Read the model definition and answer for the solid it produces. Units are mm, in the model's axes. Face numbers are marked on the shaded views. Give positions to 0.01 mm unless a question says otherwise; leave off trailing zeros. Order: outer loops, then holes, each group sorted by start corner. A loop starts at its lowest first (then second) coordinate and runs counter-clockwise, first axis right, second up. Notation, with made-up numbers: (12.25, -36) - (71.25, -36) arc R24 ccw to (71.25, -21) - close; hole circle Ø7 at (26.25, 82.5). An arc over 180 degrees is marked (long way). One line per item, written item: value. Start each with the question number.
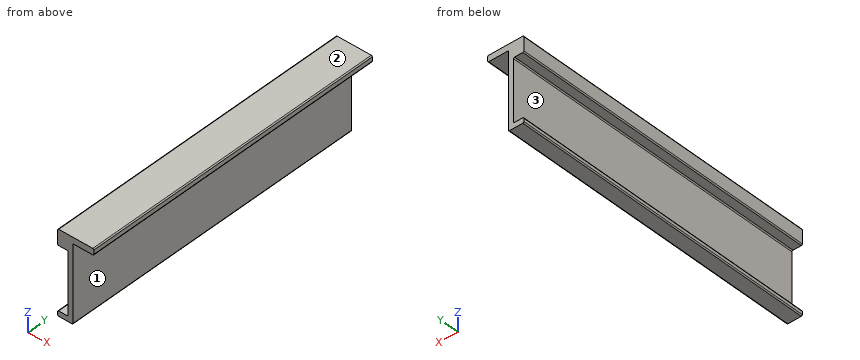
```python
from build123d import *

# Parameters (mm, degrees)
SKETCH1_W           = 300
SKETCH1_H           = 80
BOSS_EXTRUDE1_DEPTH = 15
SKETCH2_W           = 300
SKETCH2_H           = 6
BOSS_EXTRUDE2_DEPTH = 20
SKETCH3_W           = 300
SKETCH3_H           = 60
CUT_EXTRUDE1_DEPTH  = 10
FILLET1_R           = 1


with BuildPart() as part:
    # Sketch1 → Boss-Extrude1 (new body)
    with BuildSketch(Plane.YZ):
        with Locations((150, -40)):
            Rectangle(SKETCH1_W, SKETCH1_H)
    extrude(amount=BOSS_EXTRUDE1_DEPTH)

    # Sketch2 → Boss-Extrude2 (add)
    with BuildSketch(Plane.YZ.offset(15)):
        with Locations((150, -3)):
            Rectangle(SKETCH2_W, SKETCH2_H)
    extrude(amount=BOSS_EXTRUDE2_DEPTH)

    # Sketch3 → Cut-Extrude1 (cut)
    with BuildSketch(Plane(origin=(0, 0, 0), x_dir=(0, -1, 0), z_dir=(-1, 0, 0))):
        with Locations((-150, -45)):
            Rectangle(SKETCH3_W, SKETCH3_H)
    extrude(amount=-CUT_EXTRUDE1_DEPTH, mode=Mode.SUBTRACT)

    # Fillet1
    fillet1_edges = [part.edges().sort_by_distance(p)[0] for p in [
        (35, 150, -6),
        (35, 150, 0),
        (10, 150, -15),
        (10, 150, -75),
        (0, 150, -75),
        (0, 150, -15),
        (0, 150, 0),
        (0, 150, -80),
        (15, 150, -80),
    ]]
    fillet(fillet1_edges, radius=FILLET1_R)


solid = part.part
```
1) The mould has two halves that part along Z. Classify the marked faces 1, 2 and 3: +Z half, -Z half, draft (parallel to the pull), parting line (faces both ways), or undercut.
2) Section B-B on z = -37 is taken. Write down the section's boundary in (x, y), plus the area to 3 significant figures.
3) Each of these flat-tipped pins is pushed along its axis until it touches: pin 1 (12 mm diameter, centred on x = 26, y = 251, fed in from -Z); pin 2 (1 mm diameter, centred on y = 108.5, z = -12.5, fed in from +X); pin 3 (17.5 mm diameter, centred on y = 138.5, z = -37, fed in from -X). Where does it stop, or does it pass through?
4) Find the intervals of material crossed by probe 1 along Z at (x, y) = (2, 23.5); probe 2 along Z at (x, y) = (29, 93.5); probe 3 along X at (y, z) = (54, -26), in increasing order. Write a range as from..to.
5) Section A-A on y = 173 is taken. Write down the section's boundary in (x, z), plus the area to 3 significant figures.
6) Section C-C on x = 20 is taken. Write down the section's boundary in (y, z).
Solved:
1. face 1: draft
1. face 2: +Z half
1. face 3: undercut
2. outline: (10, 0) - (15, 0) - (15, 300) - (10, 300) - close
2. area: 1,500 mm2
3. pin 1: stops at z = -6
3. pin 2: stops at x = 15
3. pin 3: stops at x = 10
4. probe 1: z = -80..-75, -15..0
4. probe 2: z = -6..0
4. probe 3: x = 10..15
5. outline: (0, -79) arc R1 ccw to (1, -80) - (14, -80) arc R1 ccw to (15, -79) - (15, -6) - (34, -6) arc R1 ccw to (35, -5) - (35, -1) arc R1 ccw to (34, 0) - (1, 0) arc R1 ccw to (0, -1) - (0, -14) arc R1 ccw to (1, -15) - (9, -15) arc R1 cw to (10, -16) - (10, -74) arc R1 cw to (9, -75) - (1, -75) arc R1 ccw to (0, -76) - close
5. area: 719 mm2
6. outline: (0, -6) - (300, -6) - (300, 0) - (0, 0) - close
